Geometry check sheet. Reference: the model listing, model coordinates, mm. A direction names the side the tool comes from. Coordinates: 2 decimals unless noted, no trailing zeros. Loops run counter-clockwise (first coordinate to the right, second up) from the corner with the lowest first, then second, coordinate; pieces in that order, holes last. Notation, with made-up numbers: M 28,43.25 L 63,43.25 A25 ccw 63,64.25 Z; hole C -36.75,-36 d10. An arc over 180 degrees is marked long. One line per question, with ' | ' between items. Start each with the question number.
from build123d import *

# Parameters (mm, degrees)
BOSS_EXTRUDE1_DEPTH = 2
SKETCH2_W           = 2
SKETCH2_H           = 32
BOSS_EXTRUDE2_DEPTH = 115
SKETCH3_R           = 1.5
CUT_EXTRUDE1_DEPTH  = 127.878524582
SKETCH4_R           = 1.5875
CUT_EXTRUDE2_DEPTH  = 122.553115962


with BuildPart() as part:
    # Sketch1 → Boss-Extrude1 (new body)
    with BuildSketch(Plane(origin=(0, 0, 0), x_dir=(1, 0, 0), z_dir=(0, 1, 0))):
        Polygon((-21, 16), (-15.875, 16), (-15.875, 25.4), (15.875, 25.4), (15.875, 16), (21, 16), (21, -16), (15.875, -16), (15.875, -25.4), (-15.875, -25.4), (-15.875, -16), (-21, -16), align=None)
    extrude(amount=-BOSS_EXTRUDE1_DEPTH)

    # Sketch2 → Boss-Extrude2 (add)
    with BuildSketch(Plane.XZ.offset(2)):
        with Locations((-20, 0)):
            Rectangle(SKETCH2_W, SKETCH2_H)
        with Locations((20, 0)):
            Rectangle(SKETCH2_W, SKETCH2_H)
    extrude(amount=BOSS_EXTRUDE2_DEPTH)

    # Sketch3 → Cut-Extrude1 (cut, through all)
    with BuildSketch(Plane.ZY.offset(21)):
        with Locations((-7, -65)):
            Circle(SKETCH3_R)
        with Locations((7, -65)):
            Circle(SKETCH3_R)
        with Locations((7, -101)):
            Circle(SKETCH3_R)
        with Locations((-7, -101)):
            Circle(SKETCH3_R)
        with Locations((0, -83.336478267)):
            Circle(SKETCH3_R)
    extrude(amount=-CUT_EXTRUDE1_DEPTH, mode=Mode.SUBTRACT)

    # Sketch4 → Cut-Extrude2 (cut, through all)
    with BuildSketch(Plane(origin=(0, 0, 0), x_dir=(1, 0, 0), z_dir=(0, 1, 0))):
        with Locations(Location((-6.35, 0, 0), (0, 0, 270))):
            Circle(SKETCH4_R)
        with Locations(Location((6.35, 0, 0), (0, 0, 270))):
            Circle(SKETCH4_R)
    extrude(amount=-CUT_EXTRUDE2_DEPTH, mode=Mode.SUBTRACT)


solid = part.part
1. Sectioned sample at D-D (y = -17). Record the cut outline in (x, z), and give its area (3 significant figures).
2. Thickness scan on line 1 (Y direction, x = -20.3, z = -7); line 2 (Z direction, x = -20.2, y = -101); line 3 (X direction, y = -42.5, z = 12.5). Record the ranges inside material, lowest first.
3. Tool access check on faces 1 (the flat face through (0, -2, 0)), 2 (the cylindrical face through (4.94, -0.99, 0.73)). Record the directions out of +Z, -Z, +X, -X, +Y, -Y that give a thin tool (end or side, any length) a straight path to the whole face; none if there is none.
4. Draft check along Z on faces 3 (the cylindrical face through (-20.01, -84.67, 0.69)), 4 (the flat face through (19, -59, 0)), 5 (the flat face through (20, -54, -16)). Enter one of: +Z half, -Z half, draft (parallel to the pull), parting line (faces both ways), or undercut.
5. Depth check by flat-ended pin: pin 1 Ø0.6 at (y, z) = (-1.5, 22.5) entering from +X (3 decimals); pin 2 Ø4 at (x, y) = (19.5, -53.5) entering from -Z; pin 3 Ø2.5 at (y, z) = (-101, 7) entering from +X; pin 4 Ø4 at (x, z) = (7, 19.5) entering from -Y. Enter the tip coordinate at first touch or a pass-through.
6. Sectioned sample at C-C (x = 6.35). Record the cut outline in (y, z), and give its area (4 significant figures).
7. Sectioned sample at B-B (y = -101). Record the cut outline in (x, z), and give its area (3 significant figures).
8. Sectioned sample at A-A (z = -7). Record the cut outline in (x, y), and give its area (3 significant figures).
Result:
1) outline: M -21,-16 L -19,-16 L -19,16 L -21,16 Z; M 19,-16 L 21,-16 L 21,16 L 19,16 Z | area: 128 mm2
2) line 1: y = -117 to -102.5, -99.5 to -66.5, -63.5 to 0 | line 2: z = -16 to -8.5, -5.5 to 5.5, 8.5 to 16 | line 3: x = -21 to -19, 19 to 21
3) face 1: +Z, -Z, -Y | face 2: +Y, -Y
4) face 3: undercut | face 4: draft | face 5: -Z half
5) pin 1: stops at x = 15.875 | pin 2: stops at z = -16 | pin 3: passes through | pin 4: stops at y = -2
6) outline: M -2,-25.4 L 0,-25.4 L 0,-1.59 L -2,-1.59 Z; M -2,1.59 L 0,1.59 L 0,25.4 L -2,25.4 Z | area: 95.25 mm2
7) outline: M -21,-16 L -19,-16 L -19,-8.5 L -21,-8.5 Z; M -21,-5.5 L -19,-5.5 L -19,5.5 L -21,5.5 Z; M -21,8.5 L -19,8.5 L -19,16 L -21,16 Z; M 19,-16 L 21,-16 L 21,-8.5 L 19,-8.5 Z; M 19,-5.5 L 21,-5.5 L 21,5.5 L 19,5.5 Z; M 19,8.5 L 21,8.5 L 21,16 L 19,16 Z | area: 104 mm2
8) outline: M -21,-117 L -19,-117 L -19,-102.5 L -21,-102.5 Z; M -21,-99.5 L -19,-99.5 L -19,-66.5 L -21,-66.5 Z; M -21,-63.5 L -19,-63.5 L -19,-2 L 19,-2 L 19,-63.5 L 21,-63.5 L 21,0 L -21,0 Z; M 19,-117 L 21,-117 L 21,-102.5 L 19,-102.5 Z; M 19,-99.5 L 21,-99.5 L 21,-66.5 L 19,-66.5 Z | area: 520 mm2
